Read the model definition and answer for the solid it produces. Units are mm, in the model's axes. A direction names the side the tool comes from. Round coordinates to 2 decimals unless told otherwise and drop trailing zeros. Write each loop counter-clockwise with the first axis right and the second up, starting at its lowest first coordinate (ties: lowest second). Pieces come first, ordered by that corner, then holes. Notation, with made-up numbers: (55, 85.5) -> (71, 85.5) arc R11 ccw to (71, 106.5) -> close; hole circle Ø5 at (9.25, 46.5). An arc over 180 degrees is marked (long way). Return JSON: item names as keys, results as strings. Group by question number.
(1) A cutting plane is placed at B-B on y = 0. Give the vertices of the cut face in (x, z).
(2) Straight lines are drawn through the part: line 1 (Y direction, x = -5, z = 3.4); line 2 (Y direction, x = 7.75, z = 0.6); line 3 (X direction, y = -6, z = 3.15). For each, find the intervals that lie inside material, in ascending order.
(3) For faces 4 (the flat face through (-11, -2, 3)), 5 (the flat face through (0, 0, 6)), determine the directions among +Z, -Z, +X, -X, +Y, -Y from which every point of the face is accessible in a straight line to the end or side of a thin tool.
(4) A cutting plane is placed at C-C on z = 0.75. State how many separate pieces and enclosed holes the cut face has, then the cut area to 3 significant figures.
(5) The mould has two halves that part along Y. Classify faces 1 (the flat face through (-15, 0, 3)), 2 (the cylindrical face through (12.699, -7.715, 2.958)), 3 (the cylindrical face through (14.4, -9.43, 3.04)): released by +Y, released by -Y, zero draft, split by the parting line, or undercut.
(6) A cutting plane is placed at A-A on x = 5. Give the vertices of the cut face in (y, z).
```python
from build123d import *

# Parameters (mm, degrees)
SKETCH_1_W          = 30
SKETCH_1_H          = 20
EXTRUDE_1_DEPTH     = 6
FILLET_1_R          = 2
SKETCH_2_R          = 1.7
CUT_EXTRUDE_1_DEPTH = 20
CUT_EXTRUDE_2_DEPTH = 20
FILLET_2_R          = 1


with BuildPart() as part:
    # 草图1 → 凸台-拉伸1 (new body)
    with BuildSketch(Plane.XY):
        Rectangle(SKETCH_1_W, SKETCH_1_H)
    extrude(amount=EXTRUDE_1_DEPTH)

    # 圆角1
    fillet_1_edges = [part.edges().sort_by_distance(p)[0] for p in [
        (15, -10, 3),
        (-15, -10, 3),
        (-15, 10, 3),
        (15, 10, 3),
    ]]
    fillet(fillet_1_edges, radius=FILLET_1_R)

    # 草图2 → 切除-拉伸1 (cut, through all)
    with BuildSketch(Plane.XY.offset(6)):
        with Locations((5, 0)):
            Circle(SKETCH_2_R)
        with Locations(Location((-5, 0, 0), (0, 0, 180))):
            Circle(SKETCH_2_R)
    extrude(amount=-CUT_EXTRUDE_1_DEPTH, mode=Mode.SUBTRACT)

    # 草图3 → 切除-拉伸2 (cut, through all)
    with BuildSketch(Plane.XY.offset(6)):
        Polygon((-13, 2), (-13, 8), (-2, 8), (-2, 4), (-9, 4), (-9, 2), align=None)
        Polygon((9, 2), (13, 2), (13, 8), (2, 8), (2, 4), (9, 4), align=None)
        Polygon((13, -2), (13, -8), (2, -8), (2, -4), (9, -4), (9, -2), align=None)
        Polygon((-9, -2), (-13, -2), (-13, -8), (-2, -8), (-2, -4), (-9, -4), align=None)
    extrude(amount=-CUT_EXTRUDE_2_DEPTH, mode=Mode.SUBTRACT)

    # 圆角2
    fillet_2_edges = [part.edges().sort_by_distance(p)[0] for p in [
        (-2, -4, 3),
        (2, 8, 3),
        (13, 8, 3),
        (13, 2, 3),
        (2, 4, 3),
        (9, 2, 3),
        (9, 4, 3),
        (13, -2, 3),
        (2, -8, 3),
        (2, -4, 3),
        (9, -2, 3),
        (9, -4, 3),
        (13, -8, 3),
        (-2, -8, 3),
        (-13, -8, 3),
        (-13, -2, 3),
        (-9, -2, 3),
        (-9, -4, 3),
        (-2, 8, 3),
        (-2, 4, 3),
        (-9, 4, 3),
        (-9, 2, 3),
        (-13, 2, 3),
        (-13, 8, 3),
    ]]
    fillet(fillet_2_edges, radius=FILLET_2_R - 0.0001)  # a hair under: the kernel refuses the full size


solid = part.part
```
Checks:
{
 "1": {"outline": "(-15, 0) -> (-6.7, 0) -> (-6.7, 6) -> (-15, 6) -> close; (-3.3, 0) -> (3.3, 0) -> (3.3, 6) -> (-3.3, 6) -> close; (6.7, 0) -> (15, 0) -> (15, 6) -> (6.7, 6) -> close"},
 "2": {"line 1": "y = -10 to -8, -4 to -1.7, 1.7 to 4, 8 to 10", "line 2": "y = -10 to -8, -4 to 4, 8 to 10", "line 3": "x = -15 to -13, -2 to 2, 13 to 15"},
 "3": {"face 4": "+Z, -Z", "face 5": "+Z, +X, -X, +Y, -Y"},
 "4": {"separate pieces": "1", "enclosed holes": "6", "area": "374 mm^2"},
 "5": {"face 1": "zero draft", "face 2": "undercut", "face 3": "released by -Y"},
 "6": {"outline": "(-10, 0) -> (-8, 0) -> (-8, 6) -> (-10, 6) -> close; (-4, 0) -> (-1.7, 0) -> (-1.7, 6) -> (-4, 6) -> close; (1.7, 0) -> (4, 0) -> (4, 6) -> (1.7, 6) -> close; (8, 0) -> (10, 0) -> (10, 6) -> (8, 6) -> close"}
}
